Can you work these out from the model? Positions are in its coordinate system, mm. Face numbers are marked on the shaded views. A direction names the side the tool comes from. Give positions to 0.01 mm unless a question says otherwise; leave off trailing zeros. Order: outer loops, then holes, each group sorted by start corner. A loop starts at its lowest first (then second) coordinate and runs counter-clockwise, first axis right, second up. Notation, with made-up numbers: (-27.5, 63) - (7.5, 63) arc R14 cw to (7.5, 85) - close; hole circle Ø5 at (28.5, 3.25). An arc over 180 degrees is marked (long way). Answer as a JSON object with one key per item and string values.
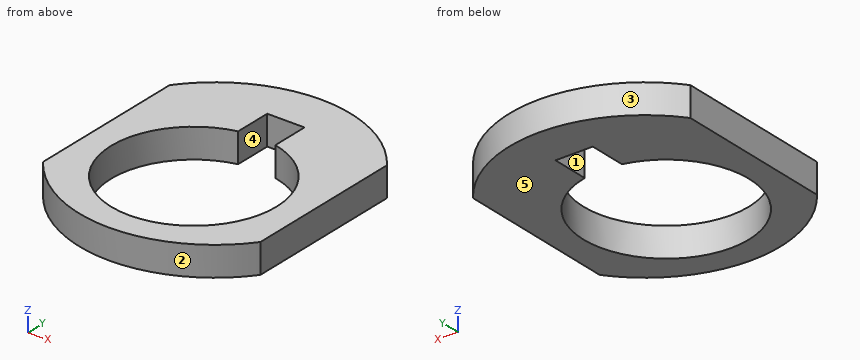
```python
from build123d import *

# Parameters (mm, degrees)
F2_DEPTH = 3


with BuildPart() as f2:
    # F1 (on Top) → F2 (new body)
    with BuildSketch(Plane.XY):
        with BuildLine():
            Line((-11.075, 8.274962), (-11.075, -8.274962))
            ThreePointArc((-11.075, -8.274962), (0, -13.825), (11.075, -8.274962))
            Line((11.075, -8.274962), (11.075, 8.274962))
            ThreePointArc((11.075, 8.274962), (0, 13.825), (-11.075, 8.274962))
        make_face()
        with BuildLine():
            ThreePointArc((1.9, 5.453852), (-0.036302, -11.174922), (-1.9, 5.462146))
            Line((-1.9, 5.462146), (-1.9, 9.262146))
            Line((-1.9, 9.262146), (1.9, 9.262146))
            Line((1.9, 9.262146), (1.9, 5.453852))
        make_face(mode=Mode.SUBTRACT)
    extrude(amount=F2_DEPTH)


solid = f2.part
```
Q1. If we section it at C-C, the plane x = 2.25: Please give me the cut outline in (y, z).
Recorded:
{"outline": "(-13.64, 0) - (-10.86, 0) - (-10.86, 3) - (-13.64, 3) - close; (5.36, 0) - (13.64, 0) - (13.64, 3) - (5.36, 3) - close"}
Q2. Which directions (+Z, -Z, +X, -X, +Y, -Y) give clear straight access to the entire face, cutting with the end or side of a thin tool? Please do the marked faces 1 and 2.
Recorded:
{"face 1": "+Z, -Z", "face 2": "+Z, -Z, -Y"}
Q3. If we section it at D-D, the plane y = 9.75: Please give me the cut outline in (x, z), then the cut area to 3 significant figures.
Recorded:
{"outline": "(-9.8, 0) - (9.8, 0) - (9.8, 3) - (-9.8, 3) - close", "area": "58.8 mm^2"}
Q4. We'd pull the mould along Y, two halves only. Please class the marked faces 3, 4 and 5: released by +Y, released by -Y, zero draft, split by the parting line, or undercut.
Recorded:
{"face 3": "released by +Y", "face 4": "undercut", "face 5": "zero draft"}
Q5. I'm going to push a flat-ended pin straight in: pin 1 Ø1 at (x, z) = (-4.5, 1.5) entering from +Y. Where does the tip first touch, or does it pass through?
Recorded:
{"pin 1": "stops at y = 13.23"}
Q6. If we section it at B-B, the plane z = 2.4: Please give me the cut outline in (x, y) (3 decimals), then the cut area to 3 significant figures.
Recorded:
{"outline": "(-11.075, -8.275) arc R13.825 ccw to (11.075, -8.275) - (11.075, 8.275) arc R13.825 ccw to (-11.075, 8.275) - close; hole (-1.9, 5.462) arc R8.425 ccw (long way) to (1.9, 5.454) - (1.9, 9.262) - (-1.9, 9.262) - close", "area": "302 mm^2"}
Q7. I need wall thicknesses on L1, parallel to X at y = 7.5, z = 0.3 (3 decimals); L2, parallel to Y at x = -1.75, z = 1.7; L3, parallel to Y at x = -7, z = 2.75. Which ranges of each line are inside material? Lowest first, please.
Recorded:
{"L1": "x = -11.075 to -1.9, 1.9 to 11.075", "L2": "y = -13.71 to -10.99, 9.26 to 13.71", "L3": "y = -11.92 to -7.46, 1.97 to 11.92"}
Q8. If we section it at A-A, the plane y = 6.5: Please give me the cut outline in (x, z) (3 decimals).
Recorded:
{"outline": "(-11.075, 0) - (-1.9, 0) - (-1.9, 3) - (-11.075, 3) - close; (1.9, 0) - (11.075, 0) - (11.075, 3) - (1.9, 3) - close"}
